from build123d import *

# Parameters (mm, degrees)
SKETCH1_R           = 15
BOSS_EXTRUDE1_DEPTH = 10
CUT_EXTRUDE1_DEPTH  = 10
CIRPATTERN1_COUNT   = 12
SKETCH3_R           = 3
CUT_EXTRUDE2_DEPTH  = 11


with BuildPart() as part:
    # Sketch1 → Boss-Extrude1 (new body)
    with BuildSketch(Plane.XY):
        Circle(SKETCH1_R)
    extrude(amount=BOSS_EXTRUDE1_DEPTH)

    # Sketch2 → Cut-Extrude1 (cut)
    with BuildSketch(Plane.XY.offset(10)):
        with BuildLine():
            Line((-2.5, 14.790199458), (-1, 11.958260743))
            ThreePointArc((-1, 11.958260743), (0, 12), (1, 11.958260743))
            Line((1, 11.958260743), (2.5, 14.790199458))
            ThreePointArc((2.5, 14.790199458), (0, 15), (-2.5, 14.790199458))
        make_face()
    cut_extrude1 = extrude(amount=-CUT_EXTRUDE1_DEPTH, mode=Mode.SUBTRACT)

    # CirPattern1: Cut-Extrude1 ×12 about axis
    cirpattern1_axis = Axis((0, 0, 0), (0, 0, 1))
    for i in range(1, CIRPATTERN1_COUNT):
        add(cut_extrude1.rotate(cirpattern1_axis, i * 360 / CIRPATTERN1_COUNT), mode=Mode.SUBTRACT)

    # Sketch3 → Cut-Extrude2 (cut, through all)
    with BuildSketch(Plane(origin=(0, 0, 0), x_dir=(-1, 0, 0), z_dir=(0, 0, -1))):
        Circle(SKETCH3_R)
    extrude(amount=-CUT_EXTRUDE2_DEPTH, mode=Mode.SUBTRACT)


solid = part.part
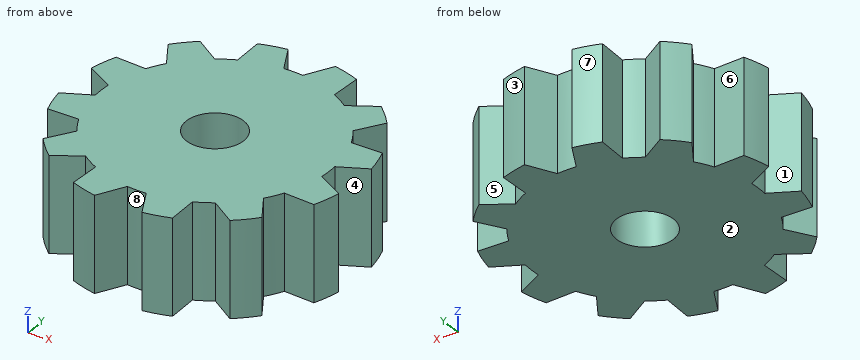
Verification items for the finished model (mm, model axes). Face numbers are marked on the shaded views. A direction names the side the tool comes from. Give positions to 0.01 mm unless a question says otherwise; leave off trailing zeros. Loops run counter-clockwise (first coordinate to the right, second up) from the corner with the lowest first, then second, coordinate; pieces in that order, holes last.
1. Tool access check on the marked faces 4, 5, 6, 7 and 8. Record the directions out of +Z, -Z, +X, -X, +Y, -Y that give a thin tool (end or side, any length) a straight path to the whole face; none if there is none.
Derived:
face 4: +Z, -Z, +X
face 5: +Z, -Z, +Y
face 6: +Z, -Z
face 7: +Z, -Z, -X, +Y
face 8: +Z, -Z, -Y
2. Go/stop test with flat-tipped pins: P1, Ø3, axis at y = -10.5, z = 7, coming from the -X side; P2, Ø2, axis at y = -11.5, z = 7, coming from the +X side; P3, Ø6, axis at x = 11.5, z = 3, coming from the -Y side. Record where each tip stops, or that it passes through.
Derived:
P1: stops at x = -11.56
P2: stops at x = 10.71
P3: stops at y = -11.56
3. Material ranges on probe 1 along X at (y, z) = (-10, 5.5); probe 2 along X at (y, z) = (2, 2.75); probe 3 along Y at (x, z) = (11.5, 3), recorded low to high.
Derived:
probe 1: x = -11.18 to -7.07, -6.63 to 6.63, 7.07 to 11.18
probe 2: x = -13.85 to -2.24, 2.24 to 13.85
probe 3: y = -9.63 to -9.47, -5.14 to 5.14, 9.47 to 9.63
4. Release check for a two-part mould opening along Y. For the marked faces 1, 2 and 3 record: +Y half, -Y half, draft (parallel to the pull), parting line (faces both ways), or undercut.
Derived:
face 1: undercut
face 2: draft
face 3: +Y half
5. Cross-section at D-D on x = 9. Record the cut outline in (y, z), and give its area (3 significant figures).
Derived:
outline: (-11.21, 0) - (11.21, 0) - (11.21, 10) - (-11.21, 10) - close
area: 224 mm2
6. Cross-section at A-A on y = 0. Record the cut outline in (x, z).
Derived:
outline: (-12, 0) - (-3, 0) - (-3, 10) - (-12, 10) - close; (3, 0) - (12, 0) - (12, 10) - (3, 10) - close
7. Cross-section at C-C on y = -7.75. Record the cut outline in (x, z).
Derived:
outline: (-10.42, 0) - (10.42, 0) - (10.42, 10) - (-10.42, 10) - close
